from build123d import *

# Parameters (mm, degrees)
SKETCH1_W           = 90
SKETCH1_H           = 61
BOSS_EXTRUDE1_DEPTH = 2
SKETCH2_W           = 90
SKETCH2_H           = 61
SKETCH2_W_2         = 86
SKETCH2_H_2         = 57
BOSS_EXTRUDE2_DEPTH = 8
SKETCH3_W           = 26
SKETCH3_H           = 7
CUT_EXTRUDE1_DEPTH  = 2
SKETCH4_W           = 2
SKETCH4_H           = 57
BOSS_EXTRUDE3_DEPTH = 4
SKETCH5_W           = 88
SKETCH5_H           = 59
SKETCH5_W_2         = 86
SKETCH5_H_2         = 57
CUT_EXTRUDE2_DEPTH  = 2


with BuildPart() as part:
    # Sketch1 → Boss-Extrude1 (new body)
    with BuildSketch(Plane(origin=(0, 0, 0), x_dir=(1, 0, 0), z_dir=(0, 1, 0))):
        with Locations((45, 30.5)):
            Rectangle(SKETCH1_W, SKETCH1_H)
    extrude(amount=BOSS_EXTRUDE1_DEPTH)

    # Sketch2 → Boss-Extrude2 (add)
    with BuildSketch(Plane(origin=(0, 2, 0), x_dir=(1, 0, 0), z_dir=(0, 1, 0))):
        with Locations((45, 30.5)):
            Rectangle(SKETCH2_W, SKETCH2_H)
        with Locations((45, 30.5)):
            Rectangle(SKETCH2_W_2, SKETCH2_H_2, mode=Mode.SUBTRACT)
    extrude(amount=BOSS_EXTRUDE2_DEPTH)

    # Sketch3 → Cut-Extrude1 (cut)
    with BuildSketch(Plane(origin=(0, 2, 0), x_dir=(1, 0, 0), z_dir=(0, 1, 0))):
        with Locations((70, 5.5)):
            Rectangle(SKETCH3_W, SKETCH3_H)
    extrude(amount=-CUT_EXTRUDE1_DEPTH, mode=Mode.SUBTRACT)

    # Sketch4 → Boss-Extrude3 (add)
    with BuildSketch(Plane(origin=(0, 2, 0), x_dir=(1, 0, 0), z_dir=(0, 1, 0))):
        with Locations((3, 30.5)):
            Rectangle(SKETCH4_W, SKETCH4_H)
        with Locations((87, 30.5)):
            Rectangle(SKETCH4_W, SKETCH4_H)
    extrude(amount=BOSS_EXTRUDE3_DEPTH)

    # Sketch5 → Cut-Extrude2 (cut)
    with BuildSketch(Plane(origin=(0, 10, 0), x_dir=(1, 0, 0), z_dir=(0, 1, 0))):
        with Locations((45, 30.5)):
            Rectangle(SKETCH5_W, SKETCH5_H)
        with Locations((45, 30.5)):
            Rectangle(SKETCH5_W_2, SKETCH5_H_2, mode=Mode.SUBTRACT)
    extrude(amount=-CUT_EXTRUDE2_DEPTH, mode=Mode.SUBTRACT)


solid = part.part
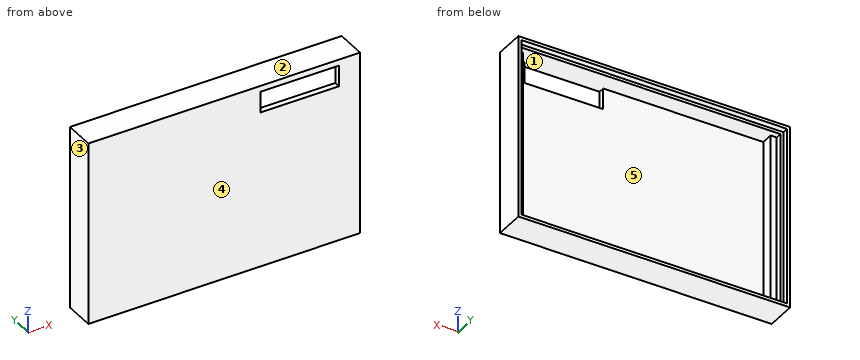
Can you work these out from the model? Positions are in its coordinate system, mm. Face numbers are marked on the shaded views. A direction names the side the tool comes from. Round coordinates to 2 decimals unless told otherwise and drop trailing zeros. Write each loop counter-clockwise with the first axis right and the second up, starting at its lowest first coordinate (ties: lowest second). Pieces come first, ordered by that corner, then holes. Notation, with made-up numbers: (-19.75, -7) -> (20.25, -7) arc R24 ccw to (20.25, 26) -> close; hole circle Ø6 at (-23.75, 45.25). An arc over 180 degrees is marked (long way). One line per question, with ' | ' between items. Start each with the question number.
1) Suppose I cut it at C-C on y = 4.75. Write out the boundary of the cut face in (x, z).
2) Suppose I cut it at B-B on x = 64.5. Write out the boundary of the cut face in (y, z).
3) If we mould it in two halves opening along X, with no side actions, what happens to the marked faces 1, 2 and 3? For each: released by +X, released by -X, zero draft, split by the parting line, or undercut.
4) I'm going to push a flat-ended pin straight in: P1, Ø1, axis at x = 87, z = -37, coming from the +Y side. Where does the tip first touch, or does it pass through?
5) Suppose I cut it at D-D on x = 39. Write out the boundary of the cut face in (y, z), then the cut area to 3 significant figures.
6) Suppose I cut it at A-A on z = -4. Write out the boundary of the cut face in (x, y), then the cut area to 3 significant figures.
7) I need wall thicknesses on line 1 (X direction, y = 5, z = -18); line 2 (X direction, y = 7.25, z = -46.5); line 3 (Z direction, x = 36, y = 8.5). Which ranges of each line are inside material? Lowest first, please. Write a range as [from, to].
8) On a 3-axis mill with a long thin cutter (end or side, diameter ignored), from which of +Z, -Z, +X, -X, +Y, -Y can I reach the whole of each face in a straight line? I mean the marked faces 4 and 5. Say none if no direction works.
Return value:
1) outline: (0, -61) -> (90, -61) -> (90, 0) -> (0, 0) -> close; hole (4, -59) -> (86, -59) -> (86, -2) -> (4, -2) -> close
2) outline: (0, -61) -> (10, -61) -> (10, -60) -> (8, -60) -> (8, -59) -> (2, -59) -> (2, -9) -> (0, -9) -> close; (0, -2) -> (8, -2) -> (8, -1) -> (10, -1) -> (10, 0) -> (0, 0) -> close
3) face 1: undercut | face 2: zero draft | face 3: released by -X
4) P1: stops at y = 6
5) outline: (0, -61) -> (10, -61) -> (10, -60) -> (8, -60) -> (8, -59) -> (2, -59) -> (2, -2) -> (8, -2) -> (8, -1) -> (10, -1) -> (10, 0) -> (0, 0) -> close | area: 150 mm2
6) outline: (0, 0) -> (57, 0) -> (57, 2) -> (4, 2) -> (4, 6) -> (2, 6) -> (2, 8) -> (1, 8) -> (1, 10) -> (0, 10) -> close; (83, 0) -> (90, 0) -> (90, 10) -> (89, 10) -> (89, 8) -> (88, 8) -> (88, 6) -> (86, 6) -> (86, 2) -> (83, 2) -> close | area: 172 mm2
7) line 1: x = [0, 4], [86, 90] | line 2: x = [0, 2], [88, 90] | line 3: z = [-61, -60], [-1, 0]
8) face 4: +Z, -Z, +X, -X, -Y | face 5: +Y
